Autodesk Inventor part; units mm, degrees
ref_plane "YZ Plane" through (0, 0, 0) normal (1, 0, 0) x (0, 1, 0)
ref_plane "XZ Plane" through (0, 0, 0) normal (0, 1, 0) x (-1, 0, 0)
ref_plane "XY Plane" through (0, 0, 0) normal (0, 0, 1) x (1, 0, 0)
sketch "Sketch1" plane through (0, 0, 0) normal (0, 1, 0) x (-1, 0, 0)
  line L0 (0, 0) -> (0, -19.05)
  circle A0 centre (0, -19.05) radius 4
  circle A1 centre (0, 0) radius 25
  dimension "d0" = 19.05
  dimension "d1" = 8
  dimension "d2" = 50
extrude "Extrusion1" add sketch "Sketch1" along normal blind 5 contours A0 | A1
sketch "Sketch2" plane through (0, 5, 0) normal (0, 1, 0) x (1, 0, 0)
  line L0 (0, 0) -> (0, 19.05)
  circle A0 centre (0, 19.05) radius 3.9
  dimension "d5" = 19.05
  dimension "d6" = 7.8
extrude "Extrusion2" add sketch "Sketch2" along normal blind 9
sketch "Sketch4" plane through (0, 5, 0) normal (0, 1, 0) x (1, 0, 0)
  circle A0 centre (0, 0) radius 9.25
  dimension "d9" = 18.5
extrude "Extrusion3" cut sketch "Sketch4" against normal blind 2
sketch "Sketch5" plane through (0, 3, 0) normal (0, 1, 0) x (1, 0, 0)
  line L0 (0, 0) -> (0, -6)
  circle A0 centre (0, -6) radius 2.125
  dimension "d12" = 6
  dimension "d13" = 4.25
extrude "Extrusion4" cut sketch "Sketch5" against normal through all
pattern_circular "Circular Pattern1" count 4 over 360 about axis through (0, 0, 0) along (0, 1, 0) of "Extrusion4"
sketch "Sketch6" plane through (0, 0, 0) normal (0, -1, 0) x (1, 0, 0)
  circle A0 centre (0, 0) radius 9
  circle A1 centre (0, 0) radius 2.125
  dimension "d19" = 18
  dimension "d20" = 4.25
extrude "Extrusion5" cut sketch "Sketch6" against normal through all contours A1
sketch "Sketch7" plane through (0, 5, 0) normal (0, 1, 0) x (1, 0, 0)
  point P0 (0, 0)
properties part number "LegWheel"
For this review, take the finished solid that the model builds, in its own axes (mm). A direction names the side the tool comes from. Give positions to 0.01 mm unless a question says otherwise; leave off trailing zeros. Order: outer loops, then holes, each group sorted by start corner. A loop starts at its lowest first (then second) coordinate and runs counter-clockwise, first axis right, second up. Notation, with made-up numbers: M 18,39 L 67,39 A18 cw 67,73 Z; hole C -29.75,-29 d5. An arc over 180 degrees is marked long. Answer in a Markdown table with one row per item. Add a question column.
(1) Consider section C-C on z = -7. State the section outline as (x, y) points (3 decimals), and give its area (3 significant figures).
(2) Mouldability with a two-part tool opening along Z and no side actions: class faces 1 (the face through (-5, 0, -5)), 2 (the face through (-0.508, 9.437, -15.183)), 3 (the face through (8.074, 1.521, 0.461)) as +Z half, -Z half, draft (parallel to the pull), parting line (faces both ways), or undercut.
(3) Consider section D-D on y = 4. State the section outline as (x, z) points, and give its area (3 significant figures).
(4) Consider section B-B on x = 6. State the section outline as (y, z) points (3 decimals).
(5) Consider section A-A on z = 0. State the section outline as (x, y) points (3 decimals), and give its area (3 significant figures).
(6) For faces 4 (the face through (-2.01, 4.01, 9.03)), 5 (the face through (0.461, 1.521, -8.074)), list the 3-axis set-ups (+Z, -Z, +X, -X, +Y, -Y) from which the entire face can be reached by the end or side of a thin tool; tool diameter is ignored.
(7) For pin 1 (10 mm diameter, centred on x = -14, z = 11, fed in from +Y); pin 2 (9 mm diameter, centred on x = 1, z = -3, fed in from +Y); pin 3 (5 mm diameter, centred on x = 1, y = 6, fed in from +Z); pin 4 (3.5 mm diameter, centred on x = -6, z = 0, fed in from -Y) (3 decimals), all flat-tipped, find the tip position at first contact; note any pin that passes through.
(8) Wall thickness on probe 1 along Z at (x, y) = (0, 1.8) (3 decimals); probe 2 along Y at (x, z) = (23, 6); probe 3 along Z at (x, y) = (-13, 2): over which ranges is each line inside the solid? List them lowest first. Write a range as [from, to].
Evaluation:
| question | item | result |
|---|---|---|
| 1 | outline | M -24,0 L -1.875,0 L -1.875,3 L -6.047,3 L -6.047,5 L -24,5 Z; M 1.875,0 L 24,0 L 24,5 L 6.047,5 L 6.047,3 L 1.875,3 Z |
| 1 | area | 205 mm^2 |
| 2 | face 1 | draft |
| 2 | face 2 | parting line |
| 2 | face 3 | undercut |
| 3 | outline | C 0,0 d50; hole C 0,0 d18.5 |
| 3 | area | 1,690 mm^2 |
| 4 | outline | M 0,-24.269 L 5,-24.269 L 5,-7.04 L 3,-7.04 L 3,-2.125 L 0,-2.125 Z; M 0,2.125 L 3,2.125 L 3,7.04 L 5,7.04 L 5,24.269 L 0,24.269 Z |
| 5 | outline | M -25,0 L -8.125,0 L -8.125,3 L -9.25,3 L -9.25,5 L -25,5 Z; M -3.875,0 L -2.125,0 L -2.125,3 L -3.875,3 Z; M 2.125,0 L 3.875,0 L 3.875,3 L 2.125,3 Z; M 8.125,0 L 25,0 L 25,5 L 9.25,5 L 9.25,3 L 8.125,3 Z |
| 5 | area | 175 mm^2 |
| 6 | face 4 | +Y |
| 6 | face 5 | +Y, -Y |
| 7 | pin 1 | stops at y = 5 |
| 7 | pin 2 | stops at y = 3 |
| 7 | pin 3 | stops at z = 25 |
| 7 | pin 4 | passes through |
| 8 | probe 1 | z = [-25, -8.125], [-3.875, -2.125], [2.125, 3.875], [8.125, 25] |
| 8 | probe 2 | y = [0, 5] |
| 8 | probe 3 | z = [-21.35, 21.35] |
